Read the model definition and answer for the solid it produces. Units are mm, in the model's axes. A direction names the side the tool comes from. Round coordinates to 2 decimals unless told otherwise and drop trailing zeros. Order: outer loops, then holes, each group sorted by start corner. A loop starts at its lowest first (then second) coordinate and runs counter-clockwise, first axis right, second up. Notation, with made-up numbers: (-11.75, 15) - (6.25, 15) arc R31 cw to (6.25, 46) - close; hole circle Ø8 at (13, 34.5). An arc over 180 degrees is marked (long way). Answer as a JSON object with one key per item and string values. Group by question number.
Q1. A cutting plane is placed at B-B on y = -0.75. Determine the outline of the cut face in (x, z).
Q2. The mould has two halves that part along Y. Classify faces 3 (the flat face through (3.53, -1.25, 7.77)), 4 (the flat face through (2, 1, 0)), 5 (the cylindrical face through (-0.41, -1.86, 2.5)): pulls with the +Y half, pulls with the -Y half, needs draft (parallel to the pull), parting line crosses it, or undercut.
Q3. A tool of negligible diameter and unlimited length cuts with its end or side. For faces 1 (the flat face through (3.53, 1.25, 7.77)), 2 (the flat face through (0, 0, 5.08)), from which of +Z, -Z, +X, -X, +Y, -Y can it reach the whole face along a straight path? Write none if from no direction.
Q4. Consider line 1 (Y direction, x = 0, z = 3.1) (3 decimals); line 2 (X direction, y = -1.1, z = 3); line 3 (X direction, y = -1.6, z = 10). Determine where each line is inside the solid, lowest interval first.
Q5. Given pin 1 Ø8 at (x, z) = (-3.5, 18) entering from -Y; pin 2 Ø1 at (y, z) = (0.5, 9) entering from -X; pin 3 Ø1.5 at (y, z) = (2, 11.5) entering from -X, each flat-ended and moving along its own axis, determine where each tip first touches the part or whether it passes through.
```python
from build123d import *

# Parameters (mm, degrees)
F1_DEPTH      = 2.54
F1_DEPTH_BACK = 2.54
F2_R          = 1.905
F3_DEPTH      = 5.08
F4_SIZE       = 2.53999


# Not quite as in the source:
# - a fillet or chamfer is up to 0.001 mm smaller than in the source, because OpenCascade refuses the exact size


with BuildPart() as f1:
    # F0 (on Front) → F1 (new body, two sides)
    with BuildSketch(Plane.XZ) as f1_sk:
        Polygon((0, 21.4385549893), (-7.62, 0), (7.62, 0), align=None)
    extrude(amount=F1_DEPTH)
    extrude(f1_sk.sketch, amount=-F1_DEPTH_BACK)

    # F2 (on Top) → F3 (cut)
    with BuildSketch(Plane.XY):
        Circle(F2_R)
    extrude(amount=F3_DEPTH, mode=Mode.SUBTRACT)

    # F4 (size 2.54 in the source; OpenCascade refuses exactly that, so slightly less here)
    f4_edges = [f1.edges().sort_by_distance(p)[0] for p in [
        (3.81, -2.54, 10.719277),
        (-3.81, -2.54, 10.719277),
        (-3.81, 2.54, 10.719277),
        (3.81, 2.54, 10.719277),
    ]]
    chamfer(f4_edges, length=F4_SIZE)


solid = f1.part
```
Result set:
{
 "1": {"outline": "(-6.82, 0) - (-1.75, 0) - (-1.75, 5.08) - (1.75, 5.08) - (1.75, 0) - (6.82, 0) - (0, 19.2) - close"},
 "2": {"face 3": "pulls with the -Y half", "face 4": "needs draft", "face 5": "undercut"},
 "3": {"face 1": "+Z, +X, +Y", "face 2": "-Z"},
 "4": {"line 1": "y = -2.54 to -1.905, 1.905 to 2.54", "line 2": "x = -5.39 to -1.56, 1.56 to 5.39", "line 3": "x = -2.37 to 2.37"},
 "5": {"pin 1": "stops at y = -1.8", "pin 2": "stops at x = -4.45", "pin 3": "stops at x = -2.25"}
}
